```python
from build123d import *

# Parameters (mm, degrees)
SKETCH1_R           = 2.45745
BOSS_EXTRUDE1_DEPTH = 2.54


with BuildPart() as part:
    # Sketch1 → Boss-Extrude1 (new body)
    with BuildSketch(Plane(origin=(0, 0, 0), x_dir=(1, 0, 0), z_dir=(0, 1, 0))):
        with BuildLine():
            Line((3.175, -4.852667781), (33.16436, -4.852667781))
            ThreePointArc((33.16436, -4.852667781), (35.40942403, -3.922731811), (36.33936, -1.677667781))
            Line((36.33936, -1.677667781), (36.33936, 54.202332219))
            ThreePointArc((36.33936, 54.202332219), (35.40942403, 56.447396249), (33.16436, 57.377332219))
            Line((33.16436, 57.377332219), (3.175, 57.377332219))
            ThreePointArc((3.175, 57.377332219), (0.92993597, 56.447396249), (0, 54.202332219))
            Line((0, 54.202332219), (0, -1.677667781))
            ThreePointArc((0, -1.677667781), (0.92993597, -3.922731811), (3.175, -4.852667781))
        make_face()
        with Locations(Location((8.89, 51.027332219, 0), (0, 0, 270))):
            Circle(SKETCH1_R, mode=Mode.SUBTRACT)
        with Locations(Location((27.94, 4.672332219, 0), (0, 0, 270))):
            Circle(SKETCH1_R, mode=Mode.SUBTRACT)
        with Locations(Location((8.89, 4.672332219, 0), (0, 0, 270))):
            Circle(SKETCH1_R, mode=Mode.SUBTRACT)
    extrude(amount=-BOSS_EXTRUDE1_DEPTH)


solid = part.part
```
Geometry: final body of the model. Coordinates: model frame, mm. Round coordinates to 2 decimals unless told otherwise and drop trailing zeros. Order: outer loops, then holes, each group sorted by start corner. A loop starts at its lowest first (then second) coordinate and runs counter-clockwise, first axis right, second up. Notation, with made-up numbers: (37, 34.5) -> (70, 34.5) arc R21 cw to (70, 70.5) -> close; hole circle Ø8 at (15.25, 81). An arc over 180 degrees is marked (long way). Use one line per item in the form item = value. Start each with the question number.
1. Line query: probe 1 along X at (y, z) = (-1.65, -4); probe 2 along Z at (x, y) = (26.5, -0.5); probe 3 along X at (y, z) = (-0.9, -3.5). Output: solid intervals per line, ascending.
2. Cut plane A-A (x = 8.89). Return the cut outline in (y, z), then the cut area to 3 significant figures.
3. Cut plane B-B (x = 27.94). Return the cut outline in (y, z).
4. Draft query along X for faces 1 (the face through (18, -1, -57.377)), 2 (the face through (9.628, -1.252, -48.683)), 3 (the face through (36.339, -1, -26)), 4 (the face through (0, -1, -27)). Return one class per face: pulls with the +X half, pulls with the -X half, needs draft (parallel to the pull), parting line crosses it, or undercut.
5. Cut plane C-C (y = -2.1). Return the cut outline in (x, z) (3 decimals), then the cut area to 3 significant figures.
6. Pin query (flat end, axial travel): pin 1 Ø4 at (x, z) = (27.94, -4.67) entering from -Y. Return the tip coordinate at first contact, or that it passes through.
Solution:
q1.probe_1 = 0 to 6.53, 11.25 to 25.58, 30.3 to 36.34
q1.probe_2 = -57.38 to -6.66, -2.68 to 4.85
q1.probe_3 = 0 to 6.73, 11.05 to 25.78, 30.1 to 36.34
q2.outline = (-2.54, -57.38) -> (0, -57.38) -> (0, -53.48) -> (-2.54, -53.48) -> close; (-2.54, -48.57) -> (0, -48.57) -> (0, -7.13) -> (-2.54, -7.13) -> close; (-2.54, -2.21) -> (0, -2.21) -> (0, 4.85) -> (-2.54, 4.85) -> close
q2.area = 133 mm^2
q3.outline = (-2.54, -57.38) -> (0, -57.38) -> (0, -7.13) -> (-2.54, -7.13) -> close; (-2.54, -2.21) -> (0, -2.21) -> (0, 4.85) -> (-2.54, 4.85) -> close
q4.face_1 = needs draft
q4.face_2 = undercut
q4.face_3 = pulls with the +X half
q4.face_4 = pulls with the -X half
q5.outline = (0, -54.202) arc R3.175 ccw to (3.175, -57.377) -> (33.164, -57.377) arc R3.175 ccw to (36.339, -54.202) -> (36.339, 1.678) arc R3.175 ccw to (33.164, 4.853) -> (3.175, 4.853) arc R3.175 ccw to (0, 1.678) -> close; hole circle Ø4.915 at (8.89, -51.027); hole circle Ø4.915 at (8.89, -4.672); hole circle Ø4.915 at (27.94, -4.672)
q5.area = 2,200 mm^2
q6.pin_1 = through
